Autodesk Inventor part; units mm, degrees
ref_plane "YZ Plane" through (0, 0, 0) normal (1, 0, 0) x (0, 1, 0)
ref_plane "XZ Plane" through (0, 0, 0) normal (0, 1, 0) x (-1, 0, 0)
ref_plane "XY Plane" through (0, 0, 0) normal (0, 0, 1) x (1, 0, 0)
sketch "Pole Base Profile" plane through (0, 0, 0) normal (0, 1, 0) x (-1, 0, 0)
  line L0 (3.5, 2.75) -> (-3.5, 2.75)
  line L1 (-3.5, 2.75) -> (-3.5, -2.75)
  line L2 (-3.5, -2.75) -> (3.5, -2.75)
  line L3 (3.5, -2.75) -> (3.5, 2.75)
  line L4 (3.5, 2.75) -> (-3.5, -2.75) construction
  line L5 (-3.5, 2.75) -> (3.5, -2.75) construction
  point P0 (0, 0)
  dimension "d0" = 7
  dimension "d1" = 5.5
extrude "Pole Base" add sketch "Pole Base Profile" along normal blind 3
sketch "Cross Base" plane through (0, 3, 0) normal (0, 1, 0) x (1, 0, 0)
  line L0 (-0.675, -2.2) -> (0.675, -2.2)
  line L1 (0.675, -2.2) -> (0.675, 2.2)
  line L2 (0.675, 2.2) -> (-0.675, 2.2)
  line L3 (-0.675, 2.2) -> (-0.675, -2.2)
  line L4 (-0.675, -2.2) -> (0.675, 2.2) construction
  line L5 (0.675, -2.2) -> (-0.675, 2.2) construction
  line L6 (-2.2, -0.675) -> (2.2, -0.675)
  line L7 (2.2, -0.675) -> (2.2, 0.675)
  line L8 (2.2, 0.675) -> (-2.2, 0.675)
  line L9 (-2.2, 0.675) -> (-2.2, -0.675)
  line L10 (-2.2, -0.675) -> (2.2, 0.675) construction
  line L11 (2.2, -0.675) -> (-2.2, 0.675) construction
  point P0 (0, 0)
  dimension "d12" = 1.35
  dimension "d13" = 4.4
  dimension "d14" = 4.4
  dimension "d15" = 1.35
extrude "Pole" add sketch "Cross Base" along normal blind 3.6
fillet "Pole Rounding" radius 0.25 8 edges at (2.2, 4.8, 0.675) (0.675, 4.8, 2.2) (-0.675, 4.8, 2.2) (-2.2, 4.8, 0.675) (-2.2, 4.8, -0.675) (-0.675, 4.8, -2.2) (0.675, 4.8, -2.2) (2.2, 4.8, -0.675)
fillet "Base Rounding" radius 0.3 4 edges at (-3.5, 3, 0) (0, 3, -2.75) (0, 3, 2.75) (3.5, 3, 0)
sketch "Top Center Point" plane through (0, 6.6, 0) normal (0, 1, 0) x (1, 0, 0)
  point P0 (0, 0)
equation "\"d0\" = s_polebl"
equation "\"d1\" = s_polebw"
equation "\"d12\" = k_cmxw"
equation "\"d13\" = k_cmxl"
equation "\"d14\" = d13"
equation "\"d15\" = d12"
equation "\"d8\" = s_poleh"
equation "\"k_width\" = 18.1"
equation "\"k_height\" = 18"
equation "\"k_taper1\" = 1.5"
equation "\"k_taper2\" = 0.5"
equation "\"k_radius\" = 6"
equation "\"k_wthick\" = 1.5"
equation "\"k_ribthick\" = 1.5"
equation "\"k_ribheight\" = 5"
equation "\"k_poleoff\" = 2.2625"
equation "\"k_poledia\" = 5.54"
equation "\"k_cmxw\" = 1.35"
equation "\"k_cmxl\" = 4.4"
equation "\"s_bwidth\" = 15.6"
equation "\"s_poleh\" = 3.6"
equation "\"s_polebw\" = 5.5"
equation "\"s_polebl\" = 7"
equation "\"b_rshift\" = 49.775"
equation "\"b_height\" = 77.4"
equation "\"b_tab\" = 27.15"
equation "\"b_lshift\" = 40.725"
equation "\"b_space\" = 117.65"
equation "\"b_caps\" = 31.675"
equation "\"b_pad\" = 1"
equation "\"b_width\" = 286.5"
equation "\"b_ctrl\" = 22.625"
equation "\"k_staper\" = 1"
equation "\"k_ltaper\" = 1.5"
equation "\"k_sradius\" = 4"
equation "\"k_lradius\" = 6"
equation "\"k_height_t\" = 16"
properties part number "keyswitch-pole_cherrymx"
Build history of the part. All positions in model axes, mm. A direction names the side the tool comes from. Give positions to 0.01 mm unless a question says otherwise; leave off trailing zeros. Loops run counter-clockwise (first coordinate to the right, second up) from the corner with the lowest first, then second, coordinate; pieces in that order, holes last. Notation, with made-up numbers: (27, 35.5) -> (40, 35.5) arc R33 cw to (40, 71.5) -> close; hole circle Ø3 at (-3, -7). An arc over 180 degrees is marked (long way). Answer in a Markdown table with one row per item.
Item 1: Tool access for faces 1 (the flat face through (-0.675, 5, -1)), 2 (the flat face through (0, 5, -2.2)), 3 (the flat face through (-1, 5, 0.675)), 4 (the flat face through (-2.2, 5, 0)), 5 (the flat face through (1, 5, -0.675)): list every direction of +Z, -Z, +X, -X, +Y, -Y with a clear straight run to the whole face (end or side of a thin tool).
Findings below:
| item | result |
|---|---|
| face 1 | -Z, -X, +Y |
| face 2 | -Z, +X, -X, +Y |
| face 3 | +Z, -X, +Y |
| face 4 | +Z, -Z, -X, +Y |
| face 5 | -Z, +X, +Y |
Item 2: Probe line 1 along Z through (x, y) = (-0.75, 5.5) (3 decimals); line 2 along X through (y, z) = (4.5, 0.3). List the from-to ranges inside material, lowest first. Write a range as [from, to].
Findings below:
| item | result |
|---|---|
| line 1 | z = [-0.675, 0.675] |
| line 2 | x = [-2.2, 2.2] |
Item 3: Slice it at A-A on y = 6. Write the cut outline in (x, z) (3 decimals), plus the area to 3 significant figures.
Findings below:
| item | result |
|---|---|
| outline | (-2.2, -0.425) arc R0.25 ccw to (-1.95, -0.675) -> (-0.675, -0.675) -> (-0.675, -1.95) arc R0.25 ccw to (-0.425, -2.2) -> (0.425, -2.2) arc R0.25 ccw to (0.675, -1.95) -> (0.675, -0.675) -> (1.95, -0.675) arc R0.25 ccw to (2.2, -0.425) -> (2.2, 0.425) arc R0.25 ccw to (1.95, 0.675) -> (0.675, 0.675) -> (0.675, 1.95) arc R0.25 ccw to (0.425, 2.2) -> (-0.425, 2.2) arc R0.25 ccw to (-0.675, 1.95) -> (-0.675, 0.675) -> (-1.95, 0.675) arc R0.25 ccw to (-2.2, 0.425) -> close |
| area | 9.95 mm² |
Item 4: Slice it at B-B on x = 1.25. Write the cut outline in (y, z) (3 decimals).
Findings below:
| item | result |
|---|---|
| outline | (0, -2.75) -> (2.7, -2.75) arc R0.3 ccw to (3, -2.45) -> (3, -0.675) -> (6.6, -0.675) -> (6.6, 0.675) -> (3, 0.675) -> (3, 2.45) arc R0.3 ccw to (2.7, 2.75) -> (0, 2.75) -> close |
Item 5: Flat gauge pins, fed straight in: P1, Ø0.9, axis at x = 0, y = 5, coming from the -Z side; P2, Ø1.4, axis at y = 5, z = -1.5, coming from the -X side (3 decimals); P3, Ø1.5, axis at y = 6, z = 0, coming from the +X side. Where does each tip first touch, or does it go through?
Findings below:
| item | result |
|---|---|
| P1 | stops at z = -2.2 |
| P2 | stops at x = -0.675 |
| P3 | stops at x = 2.2 |
Item 6: Slice it at C-C on z = -1. Write the cut outline in (x, y) (3 decimals).
Findings below:
| item | result |
|---|---|
| outline | (-3.5, 0) -> (3.5, 0) -> (3.5, 2.7) arc R0.3 ccw to (3.2, 3) -> (0.675, 3) -> (0.675, 6.6) -> (-0.675, 6.6) -> (-0.675, 3) -> (-3.2, 3) arc R0.3 ccw to (-3.5, 2.7) -> close |
Item 7: Slice it at D-D on x = 2.5. Write the cut outline in (y, z), plus the area to 3 significant figures.
Findings below:
| item | result |
|---|---|
| outline | (0, -2.75) -> (2.7, -2.75) arc R0.3 ccw to (3, -2.45) -> (3, 2.45) arc R0.3 ccw to (2.7, 2.75) -> (0, 2.75) -> close |
| area | 16.5 mm² |
